```python
from build123d import *

# Parameters (mm, degrees)
F0_W     = 50.8
F0_H     = 50.8
F1_DEPTH = 50.8
F2_R     = 10.759246


with BuildPart() as f1:
    # F0 (on Top) → F1 (new body)
    with BuildSketch(Plane.XY):
        with Locations((25.4, 25.4)):
            Rectangle(F0_W, F0_H)
    extrude(amount=F1_DEPTH)

    # F2 (on face) → F3 (revolve, cut)
    with BuildSketch(Plane.XY.offset(50.8)):
        with Locations((25.214618, 23.852944)):
            Circle(F2_R)
    revolve(axis=Axis((50.8, 25.4, 50.8), (0, 1, 0)), mode=Mode.SUBTRACT)


solid = f1.part
```
Part model, mm, in its own coordinate system. Give positions to 0.01 mm unless a question says otherwise; leave off trailing zeros. Write each loop counter-clockwise with the first axis right and the second up, starting at its lowest first coordinate (ties: lowest second). Pieces come first, ordered by that corner, then holes. Notation, with made-up numbers: M 37,-14.75 L 84,-14.75 A22 cw 84,24.25 Z; hole C 32.25,43.25 d3. An arc over 180 degrees is marked long. Use CSV: the item, a comma, the result in double quotes.
Item 1: Slice it at B-B on y = 18.5. Write the cut outline in (x, z).
Taken from the geometry:
outline,"M 0,0 L 50.8,0 L 50.8,15.88 A34.92 cw 15.88,50.8 L 0,50.8 Z; M 34.55,50.8 A16.25 ccw 50.8,34.55 L 50.8,50.8 Z"
Item 2: Drill centre lines: probe 1 along Z at (x, y) = (45, 23); probe 2 along Y at (x, z) = (37, 31); probe 3 along Y at (x, z) = (37.5, 42). Where is each one in solid material? Low to high.
Taken from the geometry:
probe 1,"z = 0 to 14.96, 37.12 to 50.8"
probe 2,"y = 0 to 13.19, 34.51 to 50.8"
probe 3,"y = 0 to 19.07, 28.64 to 50.8"
Item 3: Slice it at A-A on y = 29. Write the cut outline in (x, z).
Taken from the geometry:
outline,"M 0,0 L 50.8,0 L 50.8,15.77 A35.03 cw 15.77,50.8 L 0,50.8 Z; M 34.66,50.8 A16.14 ccw 50.8,34.66 L 50.8,50.8 Z"
